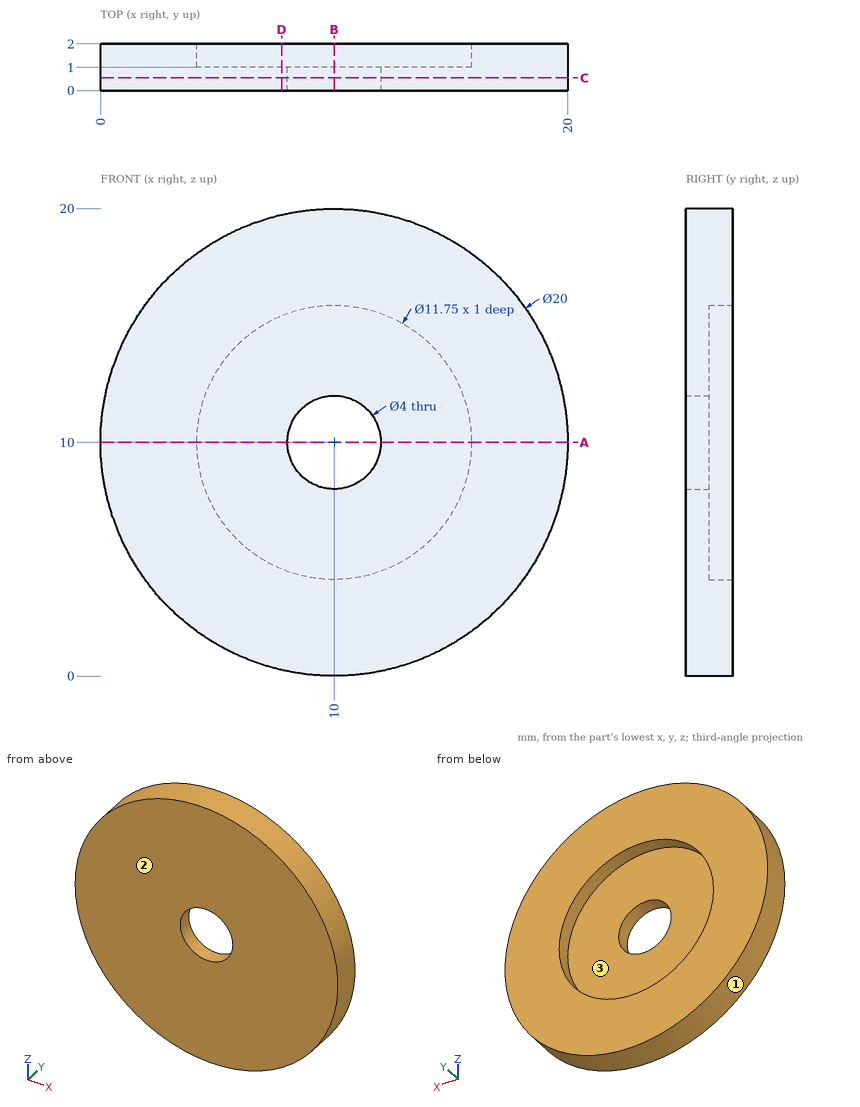
Input: dimensioned drawing with shaded views. Units: mm. Origin: part minimum x, y, z. Give positions to 0.01 mm unless a question says otherwise; leave off trailing zeros. Order: outer loops, then holes, each group sorted by start corner. A loop starts at its lowest first (then second) coordinate and runs counter-clockwise, first axis right, second up.
(1) Contact query for flat-ended pins moving along their axis: P1, Ø1, axis at x = 3.5, y = 1, coming from the +Z side; P2, Ø1, axis at x = 16, y = 0.5, coming from the +Z side. Output: stop coordinate, or through.
(2) Section query C-C (y = 0.55). Return the cut outline in (x, z).
(3) Section query D-D (x = 7.75). Return the cut outline in (y, z).
(4) Section query A-A (z = 10). Return the cut outline in (x, y) (3 decimals).
(5) Pull-direction query (X, two-part tool) for the marked faces 1, 2 and 3; classes: +X half, -X half, draft (parallel to the pull), parting line (faces both ways), or undercut.
(6) Material intervals for line 1 along Z through (x, y) = (10, 1.3) (3 decimals); line 2 along Y through (x, z) = (13.75, 6.5); line 3 along X through (y, z) = (1.45, 15), sorted ascending.
(7) Section query B-B (x = 10). Return the cut outline in (y, z) (3 decimals), plus the area to 4 significant figures.
Outcome:
1. P1: stops at z = 18
1. P2: stops at z = 18.35
2. outline: circle Ø20 at (10, 10); hole circle Ø4 at (10, 10)
3. outline: (0, 0.26) - (2, 0.26) - (2, 4.57) - (1, 4.57) - (1, 15.43) - (2, 15.43) - (2, 19.74) - (0, 19.74) - close
4. outline: (0, 0) - (8, 0) - (8, 1) - (4.125, 1) - (4.125, 2) - (0, 2) - close; (12, 0) - (20, 0) - (20, 2) - (15.875, 2) - (15.875, 1) - (12, 1) - close
5. face 1: parting line
5. face 2: draft
5. face 3: undercut
6. line 1: z = 0 to 4.125, 15.875 to 20
6. line 2: y = 0 to 1
6. line 3: x = 1.34 to 6.92, 13.08 to 18.66
7. outline: (0, 0) - (2, 0) - (2, 4.125) - (1, 4.125) - (1, 8) - (0, 8) - close; (0, 12) - (1, 12) - (1, 15.875) - (2, 15.875) - (2, 20) - (0, 20) - close
7. area: 24.25 mm2
